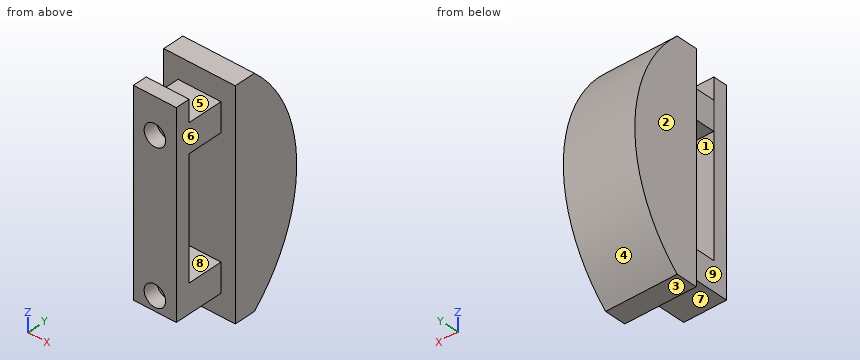
from build123d import *

# Parameters (mm, degrees)
SKETCH_1_W      = 10
SKETCH_1_H      = 30.63
EXTRUDE_1_DEPTH = 3
EXTRUDE_2_DEPTH = 10
SKETCH_3_W      = 6
SKETCH_3_H      = 4
EXTRUDE_3_DEPTH = 5
SKETCH_4_W      = 6
SKETCH_4_H      = 27.63
SKETCH_4_R      = 1.5
EXTRUDE_4_DEPTH = 2


with BuildPart() as part:
    # Эскиз1 → Бобышка-Вытянуть1 (new body)
    with BuildSketch(Plane(origin=(0, 0, 0), x_dir=(1, 0, 0), z_dir=(0, 1, 0))):
        with Locations((-87.571813581, -1.602363593)):
            Rectangle(SKETCH_1_W, SKETCH_1_H)
    extrude(amount=EXTRUDE_1_DEPTH)

    # Эскиз2 → Бобышка-Вытянуть2 (add)
    with BuildSketch(Plane(origin=(-82.571813581, 0, 0), x_dir=(0, 0, -1), z_dir=(1, 0, 0))):
        with BuildLine():
            Line((-16.917363593, 3), (13.712636407, 3))
            ThreePointArc((13.712636407, 3), (-1.602363593, 9.631604996), (-16.917363593, 3))
        make_face()
    extrude(amount=-EXTRUDE_2_DEPTH)

    # Эскиз3 → Бобышка-Вытянуть3 (add)
    with BuildSketch(Plane.XZ):
        with Locations((-87.571813581, -8.712636407)):
            Rectangle(SKETCH_3_W, SKETCH_3_H)
        Polygon((-90.562968792, 9.917363593), (-90.571813581, 13.917363593), (-84.571813581, 13.917363593), (-84.571813581, 9.917363593), align=None)
    extrude(amount=EXTRUDE_3_DEPTH)

    # Эскиз4 → Бобышка-Вытянуть4 (add)
    with BuildSketch(Plane.XZ.offset(5)):
        with Locations((-87.571813581, 3.102363593)):
            Rectangle(SKETCH_4_W, SKETCH_4_H)
        with Locations(Location((-87.571813581, 11.917363593, 0), (0, 0, 270))):
            Circle(SKETCH_4_R, mode=Mode.SUBTRACT)
        with Locations(Location((-87.571813581, -8.712636407, 0), (0, 0, 270))):
            Circle(SKETCH_4_R, mode=Mode.SUBTRACT)
    extrude(amount=EXTRUDE_4_DEPTH)


solid = part.part
Build history of the part. All positions in model axes, mm. Face numbers are marked on the shaded views. A direction names the side the tool comes from. Round coordinates to 2 decimals unless told otherwise and drop trailing zeros. Write each loop counter-clockwise with the first axis right and the second up, starting at its lowest first coordinate (ties: lowest second). Pieces come first, ordered by that corner, then holes. Notation, with made-up numbers: M 50,88.25 L 86,88.25 A10 cw 86,107.25 Z; hole C 45.25,-11 d6. An arc over 180 degrees is marked long. Use CSV: the item, a comma, the result in double quotes.
1. Saw through at D-D (x = -83.75). Give the cut face in (y, z), plus the area to 3 significant figures.
Reply:
outline,"M 0,-13.71 L 3,-13.71 A21 ccw 3,16.92 L 0,16.92 Z"
area,"232 mm²"
2. Wall check: probe 1 along Z at (x, y) = (-89, -4); probe 2 along Y at (x, z) = (-88.25, 2); probe 3 along Z at (x, y) = (-86.5, -6.5). Give the ranges that are in metal, low to high. Write a range as from..to.
Reply:
probe 1,"z = -10.71..-6.71, 9.92..13.92"
probe 2,"y = -7..-5, 0..9.63"
probe 3,"z = -10.71..-9.76, -7.66..10.87, 12.97..16.92"
3. Saw through at A-A (y = -4.5). Give the cut face in (x, z).
Reply:
outline,"M -90.57,-10.71 L -84.57,-10.71 L -84.57,-6.71 L -90.57,-6.71 Z; M -90.57,13.92 L -90.56,9.92 L -84.57,9.92 L -84.57,13.92 Z"
4. Saw through at C-C (x = -85.25). Give the cut face in (y, z).
Reply:
outline,"M -7,-10.71 L 0,-10.71 L 0,-13.71 L 3,-13.71 A21 ccw 3,16.92 L 0,16.92 L 0,13.92 L -5,13.92 L -5,16.92 L -7,16.92 Z; hole M -5,-6.71 L 0,-6.71 L 0,9.92 L -5,9.92 Z"
5. Saw through at B-B (z = 5). Give the cut face in (x, y), plus the area to 3 significant figures.
Reply:
outline,"M -92.57,0 L -82.57,0 L -82.57,9.35 L -92.57,9.35 Z; M -90.57,-7 L -84.57,-7 L -84.57,-5 L -90.57,-5 Z"
area,"106 mm²"
6. Two-plate mould, pull along Z, no slides. Class the marked faces 1, 2, 3 and 4: +Z half, -Z half, draft (parallel to the pull), parting line (faces both ways), or undercut.
Reply:
face 1,"undercut"
face 2,"draft"
face 3,"-Z half"
face 4,"parting line"
7. Flat gauge pins, fed straight in: pin 1 (1.5 mm diameter, centred on x = -87, y = -1.5, fed in from +Z); pin 2 (5 mm diameter, centred on x = -87.57, z = 11.92, fed in from +Y); pin 3 (5 mm diameter, centred on x = -88, z = 0, fed in from +Y). Where does each tip first touch, or does it go through?
Reply:
pin 1,"stops at z = 13.92"
pin 2,"stops at y = 8.12"
pin 3,"stops at y = 9.63"
8. Tool access for the marked faces 5, 6, 7, 8 and 9: list every direction of +Z, -Z, +X, -X, +Y, -Y with a clear straight run to the whole face (end or side of a thin tool).
Reply:
face 5,"+Z, +X, -X"
face 6,"+Z, -Z, +X, -Y"
face 7,"-Z, +X, -X, -Y"
face 8,"+X, -X"
face 9,"+Z, -Z, -X, -Y"
